```python
from build123d import *

# Parameters (mm, degrees)
F0_R     = 10.92
F1_DEPTH = 25.4
F2_DEPTH = 25


with BuildPart() as f1:
    # F0 (on Right) → F1 (new body)
    with BuildSketch(Plane.YZ):
        Polygon((29.540967, 29.558321), (18.013362, 37.331063), (5.518167, 31.234235), (4.550577, 17.364665), (-3.986563, 17.065152), (-4.154029, 18.255328), (-6.091229, 32.022988), (-18.982973, 37.229153), (-29.937516, 28.667658), (-28.000315, 14.899998), (-15.108572, 9.693833), (-17.46184, 1.481975), (-18.645514, 1.69049), (-32.337964, 4.102544), (-41.27309, -6.549439), (-36.515764, -19.613476), (-22.823314, -22.02553), (-13.888188, -11.373547), (-6.805447, -16.149241), (-7.369532, -17.210547), (-13.894732, -29.487476), (-6.525199, -41.276929), (7.369532, -40.789453), (13.894732, -28.512524), (6.525199, -16.723071), (13.255842, -11.462755), (14.090892, -12.327193), (23.750548, -22.326806), (37.240294, -18.961106), (41.070386, -5.595792), (31.41073, 4.403821), (17.920983, 1.03812), (14.998008, 9.064869), (16.078183, 9.591923), (28.573378, 15.688751), align=None)
        Polygon((-31.272916, 1.177826), (-20.645869, -0.694228), (-16.953593, -10.833547), (-23.888362, -19.100812), (-34.515409, -17.228758), (-38.207685, -7.089439), align=None, mode=Mode.SUBTRACT)
        Polygon((5.064367, -19.471575), (10.784042, -28.621658), (5.719675, -38.150083), (-5.064367, -38.528425), (-10.784042, -29.378342), (-5.719675, -19.849917), align=None, mode=Mode.SUBTRACT)
        Polygon((24.608011, -19.33464), (17.110916, -11.573695), (20.083544, -1.200548), (30.553267, 1.411654), (38.050362, -6.34929), (35.077734, -16.722437), align=None, mode=Mode.SUBTRACT)
        Polygon((-8.543683, 30.106279), (-7.040174, 19.42086), (-15.542264, 12.776075), (-25.547862, 16.816707), (-27.05137, 27.502125), (-18.549281, 34.146911), align=None, mode=Mode.SUBTRACT)
        Circle(F0_R, mode=Mode.SUBTRACT)
        Polygon((25.992629, 17.428877), (16.294802, 12.69698), (7.347945, 18.729595), (8.098915, 29.494108), (17.796742, 34.226006), (26.743599, 28.19339), align=None, mode=Mode.SUBTRACT)
    extrude(amount=F1_DEPTH)

    # F0 (on Right) → F2 (join)
    with BuildSketch(Plane.YZ):
        Polygon((29.540967, 29.558321), (18.013362, 37.331063), (5.518167, 31.234235), (4.550577, 17.364665), (-3.986563, 17.065152), (-4.154029, 18.255328), (-6.091229, 32.022988), (-18.982973, 37.229153), (-29.937516, 28.667658), (-28.000315, 14.899998), (-15.108572, 9.693833), (-17.46184, 1.481975), (-18.645514, 1.69049), (-32.337964, 4.102544), (-41.27309, -6.549439), (-36.515764, -19.613476), (-22.823314, -22.02553), (-13.888188, -11.373547), (-6.805447, -16.149241), (-7.369532, -17.210547), (-13.894732, -29.487476), (-6.525199, -41.276929), (7.369532, -40.789453), (13.894732, -28.512524), (6.525199, -16.723071), (13.255842, -11.462755), (14.090892, -12.327193), (23.750548, -22.326806), (37.240294, -18.961106), (41.070386, -5.595792), (31.41073, 4.403821), (17.920983, 1.03812), (14.998008, 9.064869), (16.078183, 9.591923), (28.573378, 15.688751), align=None)
        Polygon((-31.272916, 1.177826), (-20.645869, -0.694228), (-16.953593, -10.833547), (-23.888362, -19.100812), (-34.515409, -17.228758), (-38.207685, -7.089439), align=None, mode=Mode.SUBTRACT)
        Polygon((5.064367, -19.471575), (10.784042, -28.621658), (5.719675, -38.150083), (-5.064367, -38.528425), (-10.784042, -29.378342), (-5.719675, -19.849917), align=None, mode=Mode.SUBTRACT)
        Polygon((24.608011, -19.33464), (17.110916, -11.573695), (20.083544, -1.200548), (30.553267, 1.411654), (38.050362, -6.34929), (35.077734, -16.722437), align=None, mode=Mode.SUBTRACT)
        Polygon((-8.543683, 30.106279), (-7.040174, 19.42086), (-15.542264, 12.776075), (-25.547862, 16.816707), (-27.05137, 27.502125), (-18.549281, 34.146911), align=None, mode=Mode.SUBTRACT)
        Circle(F0_R, mode=Mode.SUBTRACT)
        Polygon((25.992629, 17.428877), (16.294802, 12.69698), (7.347945, 18.729595), (8.098915, 29.494108), (17.796742, 34.226006), (26.743599, 28.19339), align=None, mode=Mode.SUBTRACT)
    extrude(amount=F2_DEPTH)


solid = f1.part
```
The model under review builds one solid part; all positions refer to its coordinate system, in mm. A direction names the side the tool comes from. Round coordinates to 2 decimals unless told otherwise and drop trailing zeros. Write each loop counter-clockwise with the first axis right and the second up, starting at its lowest first coordinate (ties: lowest second). Pieces come first, ordered by that corner, then holes.
(1) We need section C-C on x = 22.75. Give the number of separate pieces and of enclosed holes in the cut face, and give its area (3 significant figures).
(2) We need section B-B on y = 0. Give the boundary of the cut face in (x, z), and give its area (3 significant figures).
(3) Insertion check: pin 1 (4 mm diameter, centred on x = 16.5, y = 6.5, fed in from +Z); pin 2 (10 mm diameter, centred on x = 17.5, y = 17, fed in from -Z); pin 3 (10 mm diameter, centred on x = 13.5, z = -13, fed in from -Y). Each pin has a flat end and moves straight along its axis. Give the tip position at first contact, or say it passes through.
(4) Mouldability with a two-part tool opening along Y and no side actions: class faces 4 (the flat face through (12.52, 29.05, 22.53)), 5 (the flat face through (12.52, 7.72, 24.04)), 6 (the flat face through (12.52, -24.38, 33.01)) as +Y half, -Y half, draft (parallel to the pull), parting line (faces both ways), or undercut.
(5) We need section A-A on y = 32.5. Give the boundary of the cut face in (x, z), and give its area (3 significant figures).
(6) Machinability: for faces 1 (the flat face through (12.52, 10.26, -22.7)), 2 (the flat face through (12.522, -38.928, -12.99)), 3 (the flat face through (12.522, 11.853, 34.325)), which of the approach directions +Z, -Z, +X, -X, +Y, -Y give a long, thin tool a straight path to every point of the face, cutting with its end or side? Answer none if there is none.
(7) Wall thickness on L1, parallel to Z at x = 19, y = 13; L2, parallel to Y at x = 17.75, z = 21.5; L3, parallel to Y at x = 4.25, z = 32.5: over which ranges is each line inside the solid? List them lowest first.
Findings below:
1. separate pieces: 1
1. enclosed holes: 6
1. area: 1,580 mm2
2. outline: (0, -41.05) - (25.4, -41.05) - (25.4, -38.35) - (0, -38.35) - close; (0, -19.65) - (25.4, -19.65) - (25.4, -10.92) - (0, -10.92) - close; (0, 10.92) - (25.4, 10.92) - (25.4, 17.21) - (0, 17.21) - close
2. area: 450 mm2
3. pin 1: stops at z = 32.69
3. pin 2: stops at z = -32.08
3. pin 3: stops at y = -40.74
4. face 4: +Y half
4. face 5: undercut
4. face 6: -Y half
5. outline: (0, -20.14) - (25.4, -20.14) - (25.4, -17.37) - (0, -17.37) - close; (0, -0.6) - (25.4, -0.6) - (25.4, 3.28) - (0, 3.28) - close
5. area: 169 mm2
6. face 1: +X, -X
6. face 2: -Z, +X, -X, -Y
6. face 3: +Z, +X, -X
7. L1: z = -30.2 to -27.08, -11.66 to 14.92, 31.89 to 34.88
7. L2: y = -28.93 to -26.21, -7.33 to -4.61, 4.84 to 7.54, 26.28 to 28.98
7. L3: y = -25.03 to -20.66, -14.47 to -7.27, 8.11 to 14.26, 20.36 to 25.18
